Read the model definition and answer for the solid it produces. Units are mm, in the model's axes. A direction names the side the tool comes from. Give positions to 0.01 mm unless a question says otherwise; leave off trailing zeros. Loops run counter-clockwise (first coordinate to the right, second up) from the corner with the lowest first, then second, coordinate; pieces in that order, holes last.
(1) Find section C-C, the plane x = -9.5. Write down the section's boundary in (y, z), then the cut area to 3 significant figures.
(2) Find section A-A, the plane y = 0. Write down the section's boundary in (x, z).
(3) Determine the mould class of faces 1 (the face through (-35, -5.3, 11.5)), 2 (the face through (-18.269, 12.932, -5.362)), 3 (the face through (-1, 0, 6)) for opening direction Z: pulls with the +Z half, pulls with the -Z half, needs draft (parallel to the pull), parting line crosses it, or undercut.
(4) Straight lines are drawn through the part: probe 1 along Z at (x, y) = (-28, 0); probe 2 along X at (y, z) = (-8, -3); probe 3 along Y at (x, z) = (-15.5, 1.25). For each, find the intervals that lie inside material, in ascending order.
(5) Each of these flat-tipped pins is pushed along its axis until it touches: P1, Ø10, axis at x = -17.5, y = 7.5, coming from the +Z side (3 decimals); P2, Ø1.5, axis at x = -24, y = -4.5, coming from the -Z side; P3, Ø1.5, axis at x = -22, z = 3, coming from the -Y side. Where does it stop, or does it pass through?
(6) Which of the six approach directions +Z, -Z, +X, -X, +Y, -Y give full straight-line access (tool end or side, diameter ignored) to faces 4 (the face through (0, -6, -2)), 5 (the face through (-19.03, 11.923, 3.755))?
Autodesk Inventor part; units mm, degrees
ref_plane "YZ Plane" through (0, 0, 0) normal (1, 0, 0) x (0, 1, 0)
ref_plane "XZ Plane" through (0, 0, 0) normal (0, 1, 0) x (-1, 0, 0)
ref_plane "XY Plane" through (0, 0, 0) normal (0, 0, 1) x (1, 0, 0)
sketch "Sketch1" plane through (0, 0, 0) normal (1, 0, 0) x (0, 1, 0)
  circle A0 centre (0, 0) radius 14
  dimension "d0" = 28
extrude "Extrusion1" add sketch "Sketch1" against normal blind 35
shell "Shell1" thickness 1.5 removed faces 1 at (-35, 2.651, 3.8406)
sketch "Sketch2" plane through (0, 0, 0) normal (1, 0, 0) x (0, 0, -1)
  point P0 (0, 0)
hole "Hole1" at (0, 0, 0) direction (-1, 0, 0) diameter 12 end through all
fillet "Fillet1" radius 2 2 edges at (0, -14, 0) (-1.5, -12.5, 0)
properties material "Steel, Mild"
Entries:
1. outline: circle Ø28 at (0, 0); hole circle Ø25 at (0, 0)
1. area: 125 mm2
2. outline: (-35, -14) - (-2, -14) arc R2 ccw to (0, -12) - (0, -6) - (-1.5, -6) - (-1.5, -10.5) arc R2 cw to (-3.5, -12.5) - (-35, -12.5) - close; (-35, 12.5) - (-3.5, 12.5) arc R2 cw to (-1.5, 10.5) - (-1.5, 6) - (0, 6) - (0, 12) arc R2 ccw to (-2, 14) - (-35, 14) - close
3. face 1: needs draft
3. face 2: parting line crosses it
3. face 3: undercut
4. probe 1: z = -14 to -12.5, 12.5 to 14
4. probe 2: x = -1.5 to 0
4. probe 3: y = -13.94 to -12.44, 12.44 to 13.94
5. P1: stops at z = 13.775
5. P2: stops at z = -13.49
5. P3: stops at y = -13.82
6. face 4: +Z, -Z, +X, +Y, -Y
6. face 5: -X
